from build123d import *

# Parameters (mm, degrees)
BOSS_EXTRUDE1_DEPTH = 100
SKETCH5_W           = 40
SKETCH5_H           = 21
CUT_EXTRUDE5_DEPTH  = 22
SKETCH3_3_R         = 2.5
CUT_EXTRUDE3_DEPTH  = 41
SKETCH3_R           = 4.25
SKETCH3_R_2         = 2.5
CUT_EXTRUDE4_DEPTH  = 6
SKETCH7_R           = 2.1
CUT_EXTRUDE7_DEPTH  = 10
SKETCH10_R          = 2.5
CUT_EXTRUDE8_DEPTH  = 3


with BuildPart() as part:
    # Sketch1 → Boss-Extrude1 (new body)
    with BuildSketch(Plane(origin=(0, 0, 0), x_dir=(1, 0, 0), z_dir=(0, 1, 0))):
        with BuildLine():
            Line((-10, -5.1), (-10, 0))
            Line((-10, 0), (-20, 0))
            Line((-20, 0), (-20, -37.5))
            Line((-20, -37.5), (-10, -37.5))
            ThreePointArc((-10, -37.5), (0, -27.5), (10, -37.5))
            Line((10, -37.5), (20, -37.5))
            Line((20, -37.5), (20, 0))
            Line((20, 0), (10, 0))
            Line((10, 0), (10, -5.1))
            Line((10, -5.1), (5.1, -5.1))
            Line((5.1, -5.1), (5.1, -15))
            Line((5.1, -15), (10.1, -15))
            Line((10.1, -15), (10.1, -20.1))
            Line((10.1, -20.1), (-10.1, -20.1))
            Line((-10.1, -20.1), (-10.1, -15))
            Line((-10.1, -15), (-5.1, -15))
            Line((-5.1, -15), (-5.1, -5.1))
            Line((-5.1, -5.1), (-10, -5.1))
        make_face()
    extrude(amount=-BOSS_EXTRUDE1_DEPTH)

    # Sketch5 → Cut-Extrude5 (cut)
    with BuildSketch(Plane.XZ.offset(100)):
        with Locations((0, 10.5)):
            Rectangle(SKETCH5_W, SKETCH5_H)
    extrude(amount=-CUT_EXTRUDE5_DEPTH, mode=Mode.SUBTRACT)

    # Sketch3_3 → Cut-Extrude3 (cut, through all)
    with BuildSketch(Plane(origin=(20, 0, 0), x_dir=(0, 0, -1), z_dir=(1, 0, 0))):
        with Locations((-10, -30)):
            Circle(SKETCH3_3_R)
    extrude(amount=-CUT_EXTRUDE3_DEPTH, mode=Mode.SUBTRACT)

    # Sketch3 → Cut-Extrude4 (cut)
    with BuildSketch(Plane(origin=(20, 0, 0), x_dir=(0, 0, -1), z_dir=(1, 0, 0))):
        with Locations((-10, -30)):
            Circle(SKETCH3_R)
        with Locations((-10, -30)):
            Circle(SKETCH3_R_2, mode=Mode.SUBTRACT)
    extrude(amount=-CUT_EXTRUDE4_DEPTH, mode=Mode.SUBTRACT)

    # Sketch7 → Cut-Extrude7 (cut)
    with BuildSketch(Plane.XY.offset(37.5)):
        with Locations((-15, -80)):
            Circle(SKETCH7_R)
        with Locations((15, -80)):
            Circle(SKETCH7_R)
        with Locations((-15, -20)):
            Circle(SKETCH7_R)
        with Locations((15, -20)):
            Circle(SKETCH7_R)
    extrude(amount=-CUT_EXTRUDE7_DEPTH, mode=Mode.SUBTRACT)

    # Sketch10 → Cut-Extrude8 (cut)
    with BuildSketch(Plane.ZY.offset(20)):
        Polygon((13.49946403, -29.9387505), (11.696688392, -26.9387505), (8.197224362, -27), (6.50053597, -30.0612495), (8.303311608, -33.0612495), (11.802775638, -33), align=None)
        with Locations((10, -30)):
            Circle(SKETCH10_R, mode=Mode.SUBTRACT)
    extrude(amount=-CUT_EXTRUDE8_DEPTH, mode=Mode.SUBTRACT)


solid = part.part
Verification items for the finished model (mm, model axes). A direction names the side the tool comes from. Give positions to 0.01 mm unless a question says otherwise; leave off trailing zeros. Write each loop counter-clockwise with the first axis right and the second up, starting at its lowest first coordinate (ties: lowest second). Pieces come first, ordered by that corner, then holes. Notation, with made-up numbers: M 43.25,73 L 83.25,73 A16 cw 83.25,81 Z; hole C -26.5,37.5 d5. An arc over 180 degrees is marked long. Put each result on its own line as item: value. Start each with the question number.
1. Section check D-D (x = 15). Record the cut outline in (y, z).
2. Go/stop test with flat-tipped pins: pin 1 Ø7.5 at (y, z) = (-30, 10) entering from +X; pin 2 Ø3 at (x, y) = (-1.5, -59.5) entering from -Z; pin 3 Ø1.5 at (x, y) = (-6.5, -27) entering from +Z. Record where each tip stops, or that it passes through.
3. Section check B-B (z = 35). Record the cut outline in (x, y).
4. Set-up check for faces 1 (the face through (-18.52, -31.54, 7.39)), 2 (the face through (17.04, -32.59, 13.37)), 3 (the face through (-16.666, -81.278, 32.57)), 4 (the face through (-10.1, -38, 18)), 5 (the face through (10, -38, 3)): record each of +Z, -Z, +X, -X, +Y, -Y from which the full face is reachable in a straight line by a thin tool's end or side.
5. Section check A-A (x = 6.5). Record the cut outline in (y, z), and give its area (3 significant figures).
6. Scan lines: line 1 along Y through (x, z) = (-15, 30); line 2 along X through (y, z) = (-43.5, 2); line 3 along X through (y, z) = (-66, 19). Record each from-to range of solid material in increasing order. Write a range as [from, to].
7. Section check C-C (y = -20). Record the cut outline in (x, z).
8. Draft check along X on faces 6 (the face through (20, -49, 19)), 7 (the face through (8, -38, 5.1)), 8 (the face through (-15, -49, 37.5)). Enter one of: +X half, -X half, draft (parallel to the pull), parting line (faces both ways), or undercut.
Answer list:
1. outline: M -100,21 L -78,21 L -78,0 L 0,0 L 0,37.5 L -17.9,37.5 L -17.9,27.5 L -22.1,27.5 L -22.1,37.5 L -77.9,37.5 L -77.9,27.5 L -82.1,27.5 L -82.1,37.5 L -100,37.5 Z; hole C -30,10 d8.5
2. pin 1: x = 14
2. pin 2: z = 20.1
2. pin 3: z = 30.61
3. outline: M -20,-100 L -9.68,-100 L -9.68,0 L -20,0 Z; M 9.68,-100 L 20,-100 L 20,0 L 9.68,0 Z; hole C -15,-80 d4.2; hole C -15,-20 d4.2; hole C 15,-80 d4.2; hole C 15,-20 d4.2
4. face 1: -X
4. face 2: +X
4. face 3: +Z
4. face 4: +Y, -Y
4. face 5: -Z, +Y, -Y
5. outline: M -100,21 L -78,21 L -78,20.1 L 0,20.1 L 0,29.9 L -100,29.9 Z; M -78,5.1 L 0,5.1 L 0,15 L -78,15 Z; hole C -30,10 d5
5. area: 1,710 mm2
6. line 1: [-100, -82.1], [-77.9, -22.1], [-17.9, 0]
6. line 2: [-20, -10], [10, 20]
6. line 3: [-20, -10.1], [10.1, 20]
7. outline: M -20,0 L -10,0 L -10,5.1 L -5.1,5.1 L -5.1,15 L -10.1,15 L -10.1,20.1 L 10.1,20.1 L 10.1,15 L 5.1,15 L 5.1,5.1 L 10,5.1 L 10,0 L 20,0 L 20,37.5 L 17.1,37.5 L 17.1,27.5 L 12.9,27.5 L 12.9,37.5 L 10,37.5 A10 cw -10,37.5 L -12.9,37.5 L -12.9,27.5 L -17.1,27.5 L -17.1,37.5 L -20,37.5 Z
8. face 6: +X half
8. face 7: undercut
8. face 8: draft
